CAD build for the part. Positions are in the model's coordinates, mm. A direction names the side the tool comes from. Round coordinates to 2 decimals unless told otherwise and drop trailing zeros. Loops run counter-clockwise (first coordinate to the right, second up) from the corner with the lowest first, then second, coordinate; pieces in that order, holes last. Notation, with made-up numbers: M 59,8 L 110,8 A34 ccw 110,42 Z; hole C 82,60.5 d11. An arc over 180 degrees is marked long. Use a Markdown table: item, result. Add a question column.
(1) Band-saw the part on A-A, the plane z = 0. Write the cut outline in (x, y).
(2) Flat gauge pins, fed straight in: P1, Ø1.5, axis at y = -6, z = -1, coming from the -X side; P2, Ø7, axis at x = 620, z = 0, coming from the -Y side; P3, Ø6, axis at x = 7, z = -0.5, coming from the -Y side; P4, Ø8, axis at x = 314, y = 5.5, coming from the -Z side. Where does each tip first touch, or does it go through?
(3) Wall check: L1, parallel to X at y = 2.3, z = 0; L2, parallel to X at y = 1.5, z = -1.5; L3, parallel to Z at x = 154.5, y = 0.25. Give the ranges that are in metal, low to high.
(4) Which spindle directions (+Z, -Z, +X, -X, +Y, -Y) get a long thin tool onto all of the face, cutting with end or side? Do faces 1 (the face through (310.59, -7.81, 1.73)), 2 (the face through (9.9, -5, -4.3)), 3 (the face through (9.9, 5, -4.3)). Say none if no direction does.
(5) Band-saw the part on B-B, the plane x = 126. Write the cut outline in (y, z), and give its area (3 significant figures).
from build123d import *

# Parameters (mm, degrees)
SKETCH_1_R               = 8
EXTRUDE_1_DEPTH          = 630
SKETCH_2_R               = 4
CUT_EXTRUDE_1_DEPTH      = 9
CUT_EXTRUDE_1_DEPTH_BACK = 9
SKETCH_3_OUTSIDE_W       = 144.082
SKETCH_3_OUTSIDE_H       = 144.082
SKETCH_3_OUTSIDE_W_2     = 20
SKETCH_3_OUTSIDE_H_2     = 10
CUT_EXTRUDE_2_DEPTH      = 20


with BuildPart() as part:
    # 草图1 → 凸台-拉伸1 (new body)
    with BuildSketch(Plane(origin=(0, 0, 0), x_dir=(0, 0, -1), z_dir=(1, 0, 0))):
        Circle(SKETCH_1_R)
    extrude(amount=EXTRUDE_1_DEPTH)

    # 草图2 → 切除-拉伸1 (cut, two sides)
    with BuildSketch(Plane(origin=(0, 0, 0), x_dir=(1, 0, 0), z_dir=(0, 1, 0))) as cut_extrude_1_sk:
        with Locations((10, 0)):
            Circle(SKETCH_2_R)
        with Locations((620, 0)):
            Circle(SKETCH_2_R)
    extrude(amount=CUT_EXTRUDE_1_DEPTH, mode=Mode.SUBTRACT)
    extrude(cut_extrude_1_sk.sketch, amount=-CUT_EXTRUDE_1_DEPTH_BACK, mode=Mode.SUBTRACT)

    # 草图3 outside → 切除-拉伸2 (cut)
    with BuildSketch(Plane.ZY):
        Rectangle(SKETCH_3_OUTSIDE_W, SKETCH_3_OUTSIDE_H)
        Rectangle(SKETCH_3_OUTSIDE_W_2, SKETCH_3_OUTSIDE_H_2, mode=Mode.SUBTRACT)
    extrude(amount=-CUT_EXTRUDE_2_DEPTH, mode=Mode.SUBTRACT)


solid = part.part
Return value:
| question | item | result |
|---|---|---|
| 1 | outline | M 0,-5 L 6,-5 L 6,5 L 0,5 Z; M 14,-5 L 20,-5 L 20,-8 L 616,-8 L 616,8 L 20,8 L 20,5 L 14,5 Z; M 624,-8 L 630,-8 L 630,8 L 624,8 Z |
| 2 | P1 | x = 20 |
| 2 | P2 | through |
| 2 | P3 | y = -5 |
| 2 | P4 | z = -7.86 |
| 3 | L1 | 0 to 6, 14 to 616, 624 to 630 |
| 3 | L2 | 0 to 6.29, 13.71 to 616.29, 623.71 to 630 |
| 3 | L3 | -8 to 8 |
| 4 | face 1 | +X, -X |
| 4 | face 2 | +Z, -Z, -X, -Y |
| 4 | face 3 | +Z, -Z, -X, +Y |
| 5 | outline | C 0,0 d16 |
| 5 | area | 201 mm^2 |
